Here's how the part is built. I have some questions about the finished solid (model axes, mm). Face numbers are marked on the shaded views. A direction names the side the tool comes from. Round coordinates to 2 decimals unless told otherwise and drop trailing zeros. Loops run counter-clockwise (first coordinate to the right, second up) from the corner with the lowest first, then second, coordinate; pieces in that order, holes last. Notation, with made-up numbers: (43, 45) - (84, 45) arc R23 ccw to (84, 57) - close; hole circle Ø2 at (13, -28.5). An arc over 180 degrees is marked (long way). Answer as a JSON object with one key per item and string values. Group by question number.
1) If I drill on line 1 along Z through (x, y) = (-20, 0.5); line 2 along Z through (x, y) = (-11.5, -24.5); line 3 along X through (y, z) = (30, 26), over which ranges is the centre line in solid material (lowest first)? Write a range as [from, to].
2) If we mould it in two halves opening along Y, with no side actions, what happens to the marked faces 1, 2, 3 and 4? For each: pulls with the +Y half, pulls with the -Y half, needs draft (parallel to the pull), parting line crosses it, or undercut.
3) I want a section at D-D, the plane x = -1.5. Please give me the cut outline in (y, z).
4) Which directions (+Z, -Z, +X, -X, +Y, -Y) give clear straight access to the entire face, cutting with the end or side of a thin tool? Please do the marked faces 5, 6, 7 and 8.
5) Will these pins go through, and if not, where does the flat tip stop? P1, Ø5, axis at y = -23, z = 52.5, coming from the +X side; P2, Ø11, axis at y = 35, z = 22.5, coming from the +X side; P3, Ø8, axis at y = 8.5, z = 42.5, coming from the +X side.
6) I want a section at C-C, the plane z = 24. Please give me the cut outline in (x, y).
7) I want a section at B-B, the plane x = 19.5. Please give me the cut outline in (y, z).
8) I want a section at A-A, the plane y = 19. Please give me the cut outline in (x, z), then the cut area to 3 significant figures.
from build123d import *

# Parameters (mm, degrees)
F0_W      = 100
F0_H      = 100
F1_DEPTH  = 15
F2_SIZE   = 12
F3_W      = 10
F3_H      = 10
F4_DEPTH  = 15
F5_W      = 10
F5_H      = 10
F6_DEPTH  = 15
F7_SIZE   = 12
F8_W      = 10
F8_H      = 10
F9_DEPTH  = 15
F10_W     = 52
F10_H     = 52
F11_DEPTH = 15
F12_SIZE  = 12
F13_DEPTH = 25
F14_SIZE  = 10


with BuildPart() as f1:
    # F0 (on Top) → F1 (new body)
    with BuildSketch(Plane.XY):
        Rectangle(F0_W, F0_H)
    extrude(amount=F1_DEPTH)

    # F2
    f2_edges = [f1.edges().sort_by_distance(p)[0] for p in [
        (0, 50, 15),
        (-50, 0, 15),
        (0, -50, 15),
        (50, 0, 15),
    ]]
    chamfer(f2_edges, length=F2_SIZE)

    # F3 (on face) → F4 (join)
    with BuildSketch(Plane.XY.offset(15)):
        with Locations((-33, 33)):
            Rectangle(F3_W, F3_H)
        with Locations((33, 33)):
            Rectangle(F3_W, F3_H)
        with Locations((33, -33)):
            Rectangle(F3_W, F3_H)
        with Locations((-33, -33)):
            Rectangle(F3_W, F3_H)
    extrude(amount=F4_DEPTH)

    # F5 (on face) → F6 (join)
    with BuildSketch(Plane.XY.offset(30)):
        Polygon((38, 38), (-28, 38), (-28, 28), (-38, 28), (-38, -38), (38, -38), align=None)
        with Locations((-33, 33)):
            Rectangle(F5_W, F5_H)
    extrude(amount=F6_DEPTH)

    # F7
    f7_edges = [f1.edges().sort_by_distance(p)[0] for p in [
        (0, 38, 45),
        (-38, 0, 45),
        (0, -38, 45),
        (38, 0, 45),
    ]]
    chamfer(f7_edges, length=F7_SIZE)

    # F8 (on face) → F9 (join)
    with BuildSketch(Plane.XY.offset(45)):
        with Locations((-21, 21)):
            Rectangle(F8_W, F8_H)
        with Locations((21, 21)):
            Rectangle(F8_W, F8_H)
        with Locations((21, -21)):
            Rectangle(F8_W, F8_H)
        with Locations((-21, -21)):
            Rectangle(F8_W, F8_H)
    extrude(amount=F9_DEPTH)

    # F10 (on face) → F11 (join)
    with BuildSketch(Plane.XY.offset(60)):
        Rectangle(F10_W, F10_H)
    extrude(amount=F11_DEPTH)

    # F12
    f12_edges = [f1.edges().sort_by_distance(p)[0] for p in [
        (0, 26, 75),
        (-26, 0, 75),
        (0, -26, 75),
        (26, 0, 75),
    ]]
    chamfer(f12_edges, length=F12_SIZE)

    # F13 (add): a face of the model
    f13_faces = [f1.faces().sort_by_distance(p)[0] for p in [
        (0, 0, 75),
    ]]
    extrude(f13_faces, amount=F13_DEPTH)

    # F14
    f14_edges = [f1.edges().sort_by_distance(p)[0] for p in [
        (0, 14, 100),
        (14, 0, 100),
        (-14, 0, 100),
        (0, -14, 100),
    ]]
    chamfer(f14_edges, length=F14_SIZE)


solid = f1.part
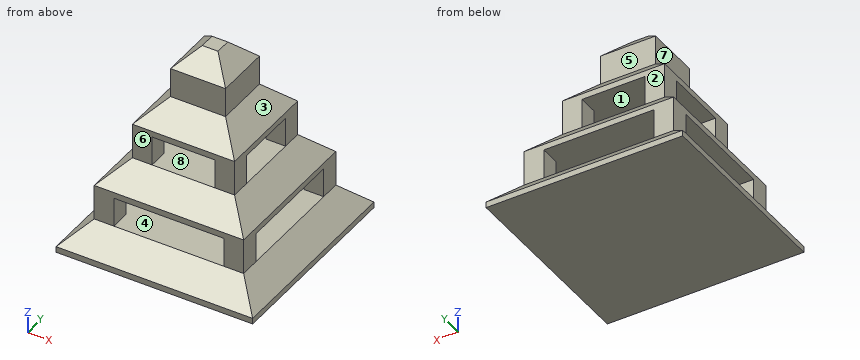
Outcome:
{
 "1": {"line 1": "[0, 15], [30, 45], [60, 69]", "line 2": "[0, 15], [30, 45], [60, 64.5]", "line 3": "[-38, -28], [28, 38]"},
 "2": {"face 1": "undercut", "face 2": "pulls with the +Y half", "face 3": "needs draft", "face 4": "undercut"},
 "3": {"outline": "(-50, 0) - (50, 0) - (50, 3) - (38, 15) - (-38, 15) - (-50, 3) - close; (-38, 30) - (38, 30) - (38, 33) - (26, 45) - (-26, 45) - (-38, 33) - close; (-26, 60) - (26, 60) - (26, 63) - (14, 75) - (14, 90) - (4, 100) - (-4, 100) - (-14, 90) - (-14, 75) - (-26, 63) - close"},
 "4": {"face 5": "+Z, +X, -X, +Y", "face 6": "+Z, +X, -X, -Y", "face 7": "+Z, -X, +Y, -Y", "face 8": "none"},
 "5": {"P1": "x = 26", "P2": "x = 38", "P3": "x = 32.5"},
 "6": {"outline": "(-38, -38) - (-28, -38) - (-28, -28) - (-38, -28) - close; (-38, 28) - (-28, 28) - (-28, 38) - (-38, 38) - close; (28, -38) - (38, -38) - (38, -28) - (28, -28) - close; (28, 28) - (38, 28) - (38, 38) - (28, 38) - close"},
 "7": {"outline": "(-50, 0) - (50, 0) - (50, 3) - (38, 15) - (-38, 15) - (-50, 3) - close; (-38, 30) - (38, 30) - (38, 33) - (26, 45) - (26, 63) - (19.5, 69.5) - (-19.5, 69.5) - (-26, 63) - (-26, 45) - (-38, 33) - close; hole (-16, 45) - (16, 45) - (16, 60) - (-16, 60) - close"},
 "8": {"outline": "(-50, 0) - (50, 0) - (50, 3) - (38, 15) - (-38, 15) - (-50, 3) - close; (-38, 30) - (38, 30) - (38, 33) - (26, 45) - (26, 63) - (19, 70) - (-19, 70) - (-26, 63) - (-26, 45) - (-38, 33) - close; hole (-16, 45) - (16, 45) - (16, 60) - (-16, 60) - close", "area": "3,120 mm^2"}
}
